Verification items for the finished model (mm, model axes). A direction names the side the tool comes from. Give positions to 0.01 mm unless a question says otherwise; leave off trailing zeros. Loops run counter-clockwise (first coordinate to the right, second up) from the corner with the lowest first, then second, coordinate; pieces in that order, holes last. Notation, with made-up numbers: (-10.75, -1) -> (25.25, -1) arc R30 cw to (25.25, 33) -> close; hole circle Ø10 at (57.25, 40.25). An arc over 180 degrees is marked (long way). Answer in a Markdown table with one row per item. Add a question column.
Q1. Set-up check for faces 1 (the face through (0, 7, 54)), 2 (the face through (-3, 38, 30)), 3 (the face through (0, 27, 60)), 4 (the face through (0, -6, 3)), 5 (the face through (3, 39, 30)): record each of +Z, -Z, +X, -X, +Y, -Y from which the full face is reachable in a straight line by a thin tool's end or side.
Q2. Material ranges on probe 1 along Y at (x, z) = (0, 2.85); probe 2 along Z at (x, y) = (4, 0); probe 3 along X at (y, z) = (21.5, 21), recorded low to high.
Q3. Release check for a two-part mould opening along X. For faces 6 (the face through (-3, 0, 3)), 7 (the face through (0, 60, 30)), 8 (the face through (0, -6, 57)) record: pulls with the +X half, pulls with the -X half, needs draft (parallel to the pull), parting line crosses it, or undercut.
Q4. Section check C-C on y = 0. Enter the section's corners in (x, z).
Q5. Section check D-D on x = -5. Enter the section's corners in (y, z).
Q6. Section check A-A on y = 14. Enter the section's corners in (x, z), and give its area (3 significant figures).
Q7. Gauge pin test, flat ends, axial feed: P1, Ø1, axis at y = 43.5, z = 38.5, coming from the -X side; P2, Ø1, axis at x = 4, y = 21.5, coming from the -Z side; P3, Ø6.5, axis at x = 0, z = 21.5, coming from the -Y side; P4, Ø4, axis at y = 21.5, z = 19, coming from the +X side. Record the tip position at first contact, or that the pin passes through.
Q8. Section check B-B on x = 0. Enter the section's corners in (y, z), and give its area (3 significant figures).
```python
from build123d import *

# Parameters (mm, degrees)
CROQUIS1_R              = 3
SALIENTE_EXTRUIR1_DEPTH = 6
CROQUIS2_W              = 6
CROQUIS2_H              = 40
SALIENTE_EXTRUIR2_DEPTH = 48
CROQUIS3_R              = 3
SALIENTE_EXTRUIR3_DEPTH = 6


with BuildPart() as part:
    # Croquis1 → Saliente-Extruir1 (new body)
    with BuildSketch(Plane.XY):
        with BuildLine():
            Line((3, 60), (-3, 60))
            Line((-3, 60), (-3, 5.196152423))
            ThreePointArc((-3, 5.196152423), (0, -6), (3, 5.196152423))
            Line((3, 5.196152423), (3, 60))
        make_face()
        Circle(CROQUIS1_R, mode=Mode.SUBTRACT)
    extrude(amount=SALIENTE_EXTRUIR1_DEPTH)

    # Croquis2 → Saliente-Extruir2 (add)
    with BuildSketch(Plane.XY.offset(6)):
        with Locations((0, 40)):
            Rectangle(CROQUIS2_W, CROQUIS2_H)
    extrude(amount=SALIENTE_EXTRUIR2_DEPTH)

    # Croquis3 → Saliente-Extruir3 (add)
    with BuildSketch(Plane.XY.offset(54)):
        with BuildLine():
            Line((-3, 5.196152423), (-3, 60))
            Line((-3, 60), (3, 60))
            Line((3, 60), (3, 5.196152423))
            ThreePointArc((3, 5.196152423), (0, -6), (-3, 5.196152423))
        make_face()
        Circle(CROQUIS3_R, mode=Mode.SUBTRACT)
    extrude(amount=SALIENTE_EXTRUIR3_DEPTH)


solid = part.part
```
Taken from the geometry:
| question | item | result |
|---|---|---|
| 1 | face 1 | +X, -X, -Y |
| 1 | face 2 | +Z, -Z, -X, +Y |
| 1 | face 3 | +Z, +X, -X, +Y, -Y |
| 1 | face 4 | +Z, -Z |
| 1 | face 5 | +Z, -Z, +X, +Y |
| 2 | probe 1 | y = -6 to -3, 3 to 60 |
| 2 | probe 2 | z = 0 to 6, 54 to 60 |
| 2 | probe 3 | x = -3 to 3 |
| 3 | face 6 | undercut |
| 3 | face 7 | needs draft |
| 3 | face 8 | parting line crosses it |
| 4 | outline | (-6, 0) -> (-3, 0) -> (-3, 6) -> (-6, 6) -> close; (-6, 54) -> (-3, 54) -> (-3, 60) -> (-6, 60) -> close; (3, 0) -> (6, 0) -> (6, 6) -> (3, 6) -> close; (3, 54) -> (6, 54) -> (6, 60) -> (3, 60) -> close |
| 5 | outline | (-3.32, 0) -> (3.32, 0) -> (3.32, 6) -> (-3.32, 6) -> close; (-3.32, 54) -> (3.32, 54) -> (3.32, 60) -> (-3.32, 60) -> close |
| 6 | outline | (-3, 0) -> (3, 0) -> (3, 6) -> (-3, 6) -> close; (-3, 54) -> (3, 54) -> (3, 60) -> (-3, 60) -> close |
| 6 | area | 72.0 mm² |
| 7 | P1 | stops at x = -3 |
| 7 | P2 | passes through |
| 7 | P3 | stops at y = 20 |
| 7 | P4 | stops at x = 3 |
| 8 | outline | (-6, 0) -> (-3, 0) -> (-3, 6) -> (-6, 6) -> close; (-6, 54) -> (-3, 54) -> (-3, 60) -> (-6, 60) -> close; (3, 0) -> (60, 0) -> (60, 60) -> (3, 60) -> (3, 54) -> (20, 54) -> (20, 6) -> (3, 6) -> close |
| 8 | area | 2,640 mm² |
